Source: CAD feature listing. Evaluate the final solid. Frame: model axes, mm. A direction names the side the tool comes from. Give positions to 0.01 mm unless a question says otherwise; leave off trailing zeros. Loops run counter-clockwise (first coordinate to the right, second up) from the corner with the lowest first, then second, coordinate; pieces in that order, holes last.
from build123d import *

# Parameters (mm, degrees)
ESTRUSIONE_ESTRUSIONE1_DEPTH = 10
SCHIZZO6_R                   = 11
TAGLIO_ESTRUSIONE4_DEPTH     = 7
SCHIZZO7_R                   = 4
TAGLIO_ESTRUSIONE5_DEPTH     = 4
SMUSSO2_SIZE                 = 10
SCHIZZO8_W                   = 20
SCHIZZO8_H                   = 4
ESTRUSIONE_ESTRUSIONE3_DEPTH = 15
SCHIZZO9_R                   = 2.5
TAGLIO_ESTRUSIONE6_DEPTH     = 35
RACCORDO1_R                  = 2
SCHIZZO10_R                  = 2.5
TAGLIO_ESTRUSIONE7_DEPTH     = 10


with BuildPart() as part:
    # Schizzo1 → Estrusione-Estrusione1 (new body)
    with BuildSketch(Plane.XY):
        Polygon((-10, -47.5), (10, -47.5), (10, -27.5), (21, -27.5), (21, 27.5), (-21, 27.5), (-21, -27.5), (-10, -27.5), align=None)
    extrude(amount=ESTRUSIONE_ESTRUSIONE1_DEPTH)

    # Schizzo6 → Taglio-Estrusione4 (cut)
    with BuildSketch(Plane.XY.offset(10)):
        Circle(SCHIZZO6_R)
    extrude(amount=-TAGLIO_ESTRUSIONE4_DEPTH, mode=Mode.SUBTRACT)

    # Schizzo7 → Taglio-Estrusione5 (cut, through all)
    with BuildSketch(Plane.XY.offset(3)):
        Circle(SCHIZZO7_R)
    extrude(amount=-TAGLIO_ESTRUSIONE5_DEPTH, mode=Mode.SUBTRACT)

    # Smusso2
    smusso2_edges = [part.edges().sort_by_distance(p)[0] for p in [
        (21, -27.5, 5),
        (-21, -27.5, 5),
        (-21, 27.5, 5),
        (21, 27.5, 5),
    ]]
    chamfer(smusso2_edges, length=SMUSSO2_SIZE)

    # Schizzo8 → Estrusione-Estrusione3 (add)
    with BuildSketch(Plane(origin=(0, 0, 0), x_dir=(-1, 0, 0), z_dir=(0, 0, -1))):
        with Locations((0, -45.5)):
            Rectangle(SCHIZZO8_W, SCHIZZO8_H)
    extrude(amount=ESTRUSIONE_ESTRUSIONE3_DEPTH)

    # Schizzo9 → Taglio-Estrusione6 (cut)
    with BuildSketch(Plane(origin=(0, -43.5, 0), x_dir=(1, 0, 0), z_dir=(0, 1, 0))):
        with Locations((0, 7.5)):
            Circle(SCHIZZO9_R)
    extrude(amount=-TAGLIO_ESTRUSIONE6_DEPTH, mode=Mode.SUBTRACT)

    # Raccordo1
    raccordo1_edges = [part.edges().sort_by_distance(p)[0] for p in [
        (0, -43.5, 0),
        (10, -45.5, -15),
        (-10, -45.5, -15),
    ]]
    fillet(raccordo1_edges, radius=RACCORDO1_R)

    # Schizzo10 → Taglio-Estrusione7 (cut)
    with BuildSketch(Plane(origin=(0, 0, 0), x_dir=(-1, 0, 0), z_dir=(0, 0, -1))):
        with Locations((0, -37.5)):
            Circle(SCHIZZO10_R)
    extrude(amount=-TAGLIO_ESTRUSIONE7_DEPTH, mode=Mode.SUBTRACT)


solid = part.part
1) Reachability of faces 1 (the flat face through (15.9, 22.6, 4.9)), 2 (the flat face through (2, -43.5, -10)), 3 (the flat face through (10, -40, 4)), 4 (the flat face through (0, -5, 3)) from +Z, -Z, +X, -X, +Y, -Y: full face, straight path, thin tool, end or side. Return the list, or none.
Checks:
face 1: +Z, -Z, +X, +Y
face 2: -Z, +X, -X, +Y
face 3: +Z, -Z, +X, -Y
face 4: +Z
2) Cut plane D-D (z = -7.5). Return loops of the section in (x, y), and give its area (3 significant figures).
Checks:
outline: (-10, -47.5) - (-2.5, -47.5) - (-2.5, -43.5) - (-10, -43.5) - close; (2.5, -47.5) - (10, -47.5) - (10, -43.5) - (2.5, -43.5) - close
area: 60.0 mm2
3) Contact query for flat-ended pins moving along their axis: P1, Ø1.5, axis at x = 6, z = -4, coming from the +Y side; P2, Ø1, axis at x = -5.5, y = 1, coming from the +Z side; P3, Ø10, axis at x = 16.5, z = 6.5, coming from the +Y side. Output: stop coordinate, or through.
Checks:
P1: stops at y = -43.5
P2: stops at z = 3
P3: stops at y = 27
4) Cut plane B-B (z = 6). Return loops of the section in (x, y).
Checks:
outline: (-21, -17.5) - (-11, -27.5) - (-10, -27.5) - (-10, -47.5) - (10, -47.5) - (10, -27.5) - (11, -27.5) - (21, -17.5) - (21, 17.5) - (11, 27.5) - (-11, 27.5) - (-21, 17.5) - close; hole circle Ø22 at (0, 0); hole circle Ø5 at (0, -37.5)
5) Ray query, probe 1 along Y at (x, z) = (1, 5.5); probe 2 along Z at (x, y) = (-6.5, 1); probe 3 along Z at (x, y) = (14.5, -17.5). Return the intervals inside material, ascending.
Checks:
probe 1: y = -47.5 to -39.79, -35.21 to -10.95, 10.95 to 27.5
probe 2: z = 0 to 3
probe 3: z = 0 to 10
6) Pull-direction query (X, two-part tool) for faces 5 (the flat face through (0, -47.5, -2)), 6 (the cylindrical face through (-2.38, -10.74, 6.55)), 7 (the cylindrical face through (0.54, -39.94, 4.93)), 8 (the flat face through (21, 0, 5)); classes: released by +X, released by -X, zero draft, split by the parting line, or undercut.
Checks:
face 5: zero draft
face 6: undercut
face 7: undercut
face 8: released by +X
7) Cut plane A-A (x = 0). Return loops of the section in (y, z), and give its area (3 significant figures).
Checks:
outline: (-47.5, -15) - (-43.5, -15) - (-43.5, -10) - (-47.5, -10) - close; (-47.5, -5) - (-43.5, -5) - (-43.5, -2) arc R2 cw to (-41.5, 0) - (-40, 0) - (-40, 10) - (-47.5, 10) - close; (-35, 0) - (-4, 0) - (-4, 3) - (-11, 3) - (-11, 10) - (-35, 10) - close; (4, 0) - (27.5, 0) - (27.5, 10) - (11, 10) - (11, 3) - (4, 3) - close
area: 563 mm2
8) Cut plane C-C (y = 0). Return loops of the section in (x, z), and give its area (3 significant figures).
Checks:
outline: (-21, 0) - (-4, 0) - (-4, 3) - (-11, 3) - (-11, 10) - (-21, 10) - close; (4, 0) - (21, 0) - (21, 10) - (11, 10) - (11, 3) - (4, 3) - close
area: 242 mm2
